from build123d import *

# Parameters (mm, degrees)
F1_DEPTH      = 57.404
F1_DEPTH_BACK = 64.516
F2_T          = -25.4


with BuildPart() as f1:
    # F0 (on Top) → F1 (new body, two sides)
    with BuildSketch(Plane.XY) as f1_sk:
        Polygon((127, 25.4), (-101.6, 25.4), (-13.6118189755, -127), (39.0118189755, -127), align=None)
    extrude(amount=-F1_DEPTH)
    extrude(f1_sk.sketch, amount=F1_DEPTH_BACK)

    # F2
    f2_openings = [f1.faces().sort_by_distance(p)[0] for p in [
        (12.7, -34.905889, 64.516),
        (12.7, -34.905889, -57.404),
        (-57.605909, -50.8, 3.556),
    ]]
    offset(amount=F2_T, openings=f2_openings)


solid = f1.part
Source: CAD feature listing. Evaluate the final solid. Frame: model axes, mm. A direction names the side the tool comes from. Coordinates: 2 decimals unless noted, no trailing zeros. Loops run counter-clockwise (first coordinate to the right, second up) from the corner with the lowest first, then second, coordinate; pieces in that order, holes last. Notation, with made-up numbers: (-21.5, 42) - (35.5, 42) arc R37 cw to (35.5, 79) - close; hole circle Ø10 at (88.25, 83). An arc over 180 degrees is marked (long way). Return JSON: item names as keys, results as strings.
Q1. Section C-C, the plane x = -81. Return loops of the section in (y, z).
Results:
{"outline": "(0, -57.4) - (25.4, -57.4) - (25.4, 64.52) - (0, 64.52) - close"}
Q2. Mould query, pull axis Y, two halves, no side actions, for faces 3 (the flat face through (14, 25.4, 3)), 4 (the flat face through (-2, -101.6, 3)), 5 (the flat face through (12, -127, 3)), 6 (the flat face through (29.1, 0.4, -57.404)). Classes: released by +Y, released by -Y, zero draft, split by the parting line, or undercut.
Results:
{"face 3": "released by +Y", "face 4": "undercut", "face 5": "released by -Y", "face 6": "zero draft"}
Q3. Access query for faces 1 (the flat face through (-1, 0, 3)), 2 (the flat face through (29.1, 0.4, 64.516)). Directions: +Z, -Z, +X, -X, +Y, -Y. A direction counts if a zero-diameter tool reaches every point of the face in a straight line with its end or side. Return the directions, or none.
Results:
{"face 1": "+Z, -Z, -X", "face 2": "+Z, +X, -X, +Y, -Y"}
Q4. Material intervals for line 1 along Y through (x, z) = (10, -18.5); line 2 along Y through (x, z) = (-64.5, 9); line 3 along Y through (x, z) = (79.5, -29), sorted ascending.
Results:
{"line 1": "-127 to -101.6, 0 to 25.4", "line 2": "0 to 25.4", "line 3": "-56.87 to -6.07, 0 to 25.4"}
Q5. Section D-D, the plane y = -48. Return loops of the section in (x, z), plus the area to 3 significant figures.
Results:
{"outline": "(55.29, -57.4) - (84.62, -57.4) - (84.62, 64.52) - (55.29, 64.52) - close", "area": "3,580 mm2"}
Q6. Section B-B, the plane x = 53. Return loops of the section in (y, z).
Results:
{"outline": "(-102.77, -57.4) - (-51.97, -57.4) - (-51.97, 64.52) - (-102.77, 64.52) - close; (0, -57.4) - (25.4, -57.4) - (25.4, 64.52) - (0, 64.52) - close"}
Q7. Section A-A, the plane z = -12. Return loops of the section in (x, y), plus the area to 3 significant figures.
Results:
{"outline": "(-101.6, 25.4) - (-86.94, 0) - (83.01, 0) - (24.35, -101.6) - (-28.28, -101.6) - (-13.61, -127) - (39.01, -127) - (127, 25.4) - close", "area": "10,100 mm2"}
Q8. Contact query for flat-ended pins moving along their axis: P1, Ø10, axis at y = -34.5, z = -6, coming from the +X side; P2, Ø4, axis at y = -49.5, z = 35, coming from the -X side; P3, Ø1.5, axis at y = -94.5, z = 43, coming from the -X side. Output: stop coordinate, or through.
Results:
{"P1": "x = 95.3", "P2": "x = 53.27", "P3": "x = 28.01"}
